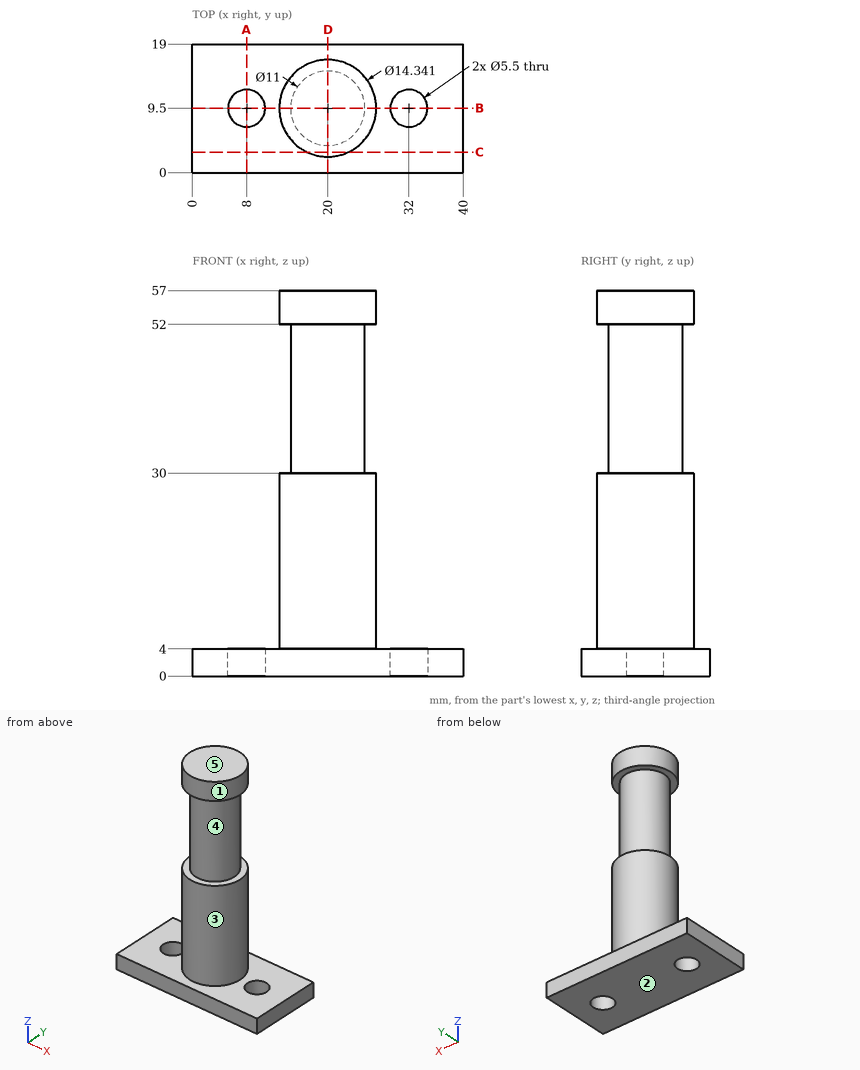
Part print with two shaded views. Sizes in mm from the minimum x, y, z corner. A direction names the side the tool comes from. Round coordinates to 2 decimals unless told otherwise and drop trailing zeros. Order: outer loops, then holes, each group sorted by start corner. A loop starts at its lowest first (then second) coordinate and runs counter-clockwise, first axis right, second up.
(1) Drill centre lines: line 1 (Y direction, x = 8, z = 1.4); line 2 (Z direction, x = 3.5, y = 2.25); line 3 (Y direction, x = 25, z = 38). Where is each one in solid material? Low to high.
(2) Band-saw the part on B-B (y = 9.5). List the corners of the cut face in (x, z), then the cut area to 3 significant figures.
(3) Band-saw the part on D-D (x = 20). List the corners of the cut face in (y, z).
(4) 3-axis set-ups, long thin cutter, end or side, ignore diameter. For the marked faces 1 and 2: which of +Z, -Z, +X, -X, +Y, -Y reach the whole face in a straight line?
(5) Band-saw the part on C-C (y = 3). List the corners of the cut face in (x, z), then the cut area to 3 significant figures.
(6) Pull direction Z, two halves, no side cores. Call the marked faces 3, 4 and 5: released by +Z, released by -Z, zero draft, split by the parting line, or undercut.
(7) Pin check, flat tips, straight feed: pin 1 (9.5 mm diameter, centred on x = 26, y = 14, fed in from +Z); pin 2 (2 mm diameter, centred on y = 16, z = 11.5, fed in from +X); pin 3 (6 mm diameter, centred on y = 8.5, z = 38.5, fed in from +X); pin 4 (8 mm diameter, centred on y = 10, z = 24, fed in from -X). Stop position of each tip, or through.
(8) Band-saw the part on A-A (x = 8). List the corners of the cut face in (y, z), then the cut area to 3 significant figures.
Verdict:
1. line 1: y = 0 to 6.75, 12.25 to 19
1. line 2: z = 0 to 4
1. line 3: y = 7.21 to 11.79
2. outline: (0, 0) - (5.25, 0) - (5.25, 4) - (0, 4) - close; (10.75, 0) - (29.25, 0) - (29.25, 4) - (27.17, 4) - (27.17, 30) - (25.5, 30) - (25.5, 52) - (27.17, 52) - (27.17, 57) - (12.83, 57) - (12.83, 52) - (14.5, 52) - (14.5, 30) - (12.83, 30) - (12.83, 4) - (10.75, 4) - close; (34.75, 0) - (40, 0) - (40, 4) - (34.75, 4) - close
2. area: 803 mm2
3. outline: (0, 0) - (19, 0) - (19, 4) - (16.67, 4) - (16.67, 30) - (15, 30) - (15, 52) - (16.67, 52) - (16.67, 57) - (2.33, 57) - (2.33, 52) - (4, 52) - (4, 30) - (2.33, 30) - (2.33, 4) - (0, 4) - close
4. face 1: +Z
4. face 2: -Z, +X, -X, +Y, -Y
5. outline: (0, 0) - (40, 0) - (40, 4) - (23.03, 4) - (23.03, 30) - (16.97, 30) - (16.97, 4) - (0, 4) - close; (16.97, 52) - (23.03, 52) - (23.03, 57) - (16.97, 57) - close
5. area: 348 mm2
6. face 3: zero draft
6. face 4: undercut
6. face 5: released by +Z
7. pin 1: stops at z = 57
7. pin 2: stops at x = 24.6
7. pin 3: stops at x = 25.5
7. pin 4: stops at x = 12.83
8. outline: (0, 0) - (6.75, 0) - (6.75, 4) - (0, 4) - close; (12.25, 0) - (19, 0) - (19, 4) - (12.25, 4) - close
8. area: 54.0 mm2
